For this review, take the finished solid that the model builds, in its own axes (mm). Coordinates: 2 decimals unless noted, no trailing zeros. Order: outer loops, then holes, each group sorted by start corner. A loop starts at its lowest first (then second) coordinate and runs counter-clockwise, first axis right, second up. Notation, with made-up numbers: (45.25, -16) -> (92.25, -16) arc R17 cw to (92.25, -7) -> close; hole circle Ø2 at (-13.5, 9.25). An arc over 180 degrees is marked (long way). Answer as a JSON object with one key per item and string values. Group by question number.
1) Wall thickness on L1, parallel to Y at x = 218, z = 0.9; L2, parallel to Y at x = 115, z = 1.25; L3, parallel to Y at x = 76.5, z = 1.25: over which ranges is each line inside the solid? List them lowest first.
2) Add section A-A, the plane y = 203.5. Write out the cut boundary in (x, z).
3) For pin 1 (3.5 mm diameter, centred on x = 111, y = 10.5, fed in from +Z), flat-tipped, find the tip position at first contact; note if it passes through.
4) Add section B-B, the plane z = 1.05. Count the separate pieces of the cut face and the enclosed holes in it, then the cut area to 3 significant figures.
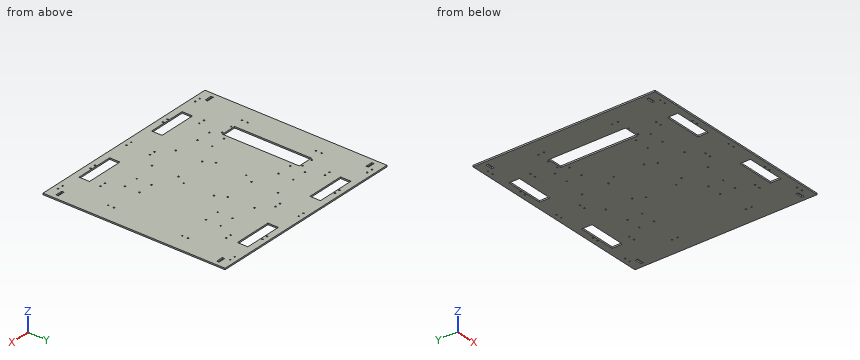
from build123d import *

# Parameters (mm, degrees)
SKETCH_1_W          = 424
SKETCH_1_H          = 384
SKETCH_1_W_2        = 80
SKETCH_1_H_2        = 22
EXTRUDE_1_DEPTH     = 3
SKETCH_2_R          = 1.5
SKETCH_2_W          = 32
SKETCH_2_H          = 162
CUT_EXTRUDE_1_DEPTH = 573.049823005
SKETCH_3_R          = 1.5
CUT_EXTRUDE_2_DEPTH = 573.049823005
SKETCH_4_R          = 1.5
CUT_EXTRUDE_3_DEPTH = 573.049823005
SKETCH_5_W          = 15
SKETCH_5_H          = 5
CUT_EXTRUDE_4_DEPTH = 573.049823005
SKETCH_6_R          = 1.5
CUT_EXTRUDE_5_DEPTH = 573.049823005


with BuildPart() as part:
    # 草图1 → 凸台-拉伸1 (new body)
    with BuildSketch(Plane.XY):
        with Locations((212, 192)):
            Rectangle(SKETCH_1_W, SKETCH_1_H)
        with Locations((307, 359)):
            Rectangle(SKETCH_1_W_2, SKETCH_1_H_2, mode=Mode.SUBTRACT)
        with Locations((117, 359)):
            Rectangle(SKETCH_1_W_2, SKETCH_1_H_2, mode=Mode.SUBTRACT)
        with Locations((307, 25)):
            Rectangle(SKETCH_1_W_2, SKETCH_1_H_2, mode=Mode.SUBTRACT)
        with Locations((117, 25)):
            Rectangle(SKETCH_1_W_2, SKETCH_1_H_2, mode=Mode.SUBTRACT)
    extrude(amount=EXTRUDE_1_DEPTH)

    # 草图2 → 切除-拉伸1 (cut, through all)
    with BuildSketch(Plane.XY.offset(3)):
        with Locations((64, 277)):
            Circle(SKETCH_2_R)
        with Locations((88, 277)):
            Circle(SKETCH_2_R)
        with Locations(Location((88, 107, 0), (0, 0, 180))):
            Circle(SKETCH_2_R)
        with Locations(Location((64, 107, 0), (0, 0, 180))):
            Circle(SKETCH_2_R)
        with Locations((76, 192)):
            Rectangle(SKETCH_2_W, SKETCH_2_H)
    extrude(amount=-CUT_EXTRUDE_1_DEPTH, mode=Mode.SUBTRACT)

    # 草图3 → 切除-拉伸2 (cut, through all)
    with BuildSketch(Plane.XY.offset(3)):
        with Locations((101.5, 293)):
            Circle(SKETCH_3_R)
        with Locations((132.5, 293)):
            Circle(SKETCH_3_R)
        with Locations((101.5, 262)):
            Circle(SKETCH_3_R)
        with Locations((132.5, 262)):
            Circle(SKETCH_3_R)
        with Locations(Location((322.5, 262, 0), (0, 0, 180))):
            Circle(SKETCH_3_R)
        with Locations(Location((291.5, 262, 0), (0, 0, 180))):
            Circle(SKETCH_3_R)
        with Locations(Location((291.5, 293, 0), (0, 0, 180))):
            Circle(SKETCH_3_R)
        with Locations(Location((322.5, 293, 0), (0, 0, 180))):
            Circle(SKETCH_3_R)
        with Locations((291.5, 122)):
            Circle(SKETCH_3_R)
        with Locations((322.5, 122)):
            Circle(SKETCH_3_R)
        with Locations((322.5, 91)):
            Circle(SKETCH_3_R)
        with Locations((291.5, 91)):
            Circle(SKETCH_3_R)
        with Locations(Location((101.5, 122, 0), (0, 0, 180))):
            Circle(SKETCH_3_R)
        with Locations(Location((132.5, 122, 0), (0, 0, 180))):
            Circle(SKETCH_3_R)
        with Locations(Location((132.5, 91, 0), (0, 0, 180))):
            Circle(SKETCH_3_R)
        with Locations(Location((101.5, 91, 0), (0, 0, 180))):
            Circle(SKETCH_3_R)
    extrude(amount=-CUT_EXTRUDE_2_DEPTH, mode=Mode.SUBTRACT)

    # 草图4 → 切除-拉伸3 (cut, through all)
    with BuildSketch(Plane.XY.offset(3)):
        with Locations((218, 10.5)):
            Circle(SKETCH_4_R)
        with Locations((301, 10.5)):
            Circle(SKETCH_4_R)
        with Locations((313, 10.5)):
            Circle(SKETCH_4_R)
        with Locations((385.5, 10.5)):
            Circle(SKETCH_4_R)
        with Locations((397.5, 10.5)):
            Circle(SKETCH_4_R)
        with Locations((218, 59.5)):
            Circle(SKETCH_4_R)
        with Locations((335.5, 59.5)):
            Circle(SKETCH_4_R)
        with Locations((347.5, 59.5)):
            Circle(SKETCH_4_R)
        with Locations((387, 108)):
            Circle(SKETCH_4_R)
        with Locations((387, 120)):
            Circle(SKETCH_4_R)
        with Locations(Location((387, 276, 0), (0, 0, 180))):
            Circle(SKETCH_4_R)
        with Locations(Location((387, 264, 0), (0, 0, 180))):
            Circle(SKETCH_4_R)
        with Locations(Location((301, 373.5, 0), (0, 0, 180))):
            Circle(SKETCH_4_R)
        with Locations(Location((313, 373.5, 0), (0, 0, 180))):
            Circle(SKETCH_4_R)
        with Locations(Location((397.5, 373.5, 0), (0, 0, 180))):
            Circle(SKETCH_4_R)
        with Locations(Location((385.5, 373.5, 0), (0, 0, 180))):
            Circle(SKETCH_4_R)
        with Locations(Location((347.5, 324.5, 0), (0, 0, 180))):
            Circle(SKETCH_4_R)
        with Locations(Location((335.5, 324.5, 0), (0, 0, 180))):
            Circle(SKETCH_4_R)
        with Locations(Location((218, 373.5, 0), (0, 0, 180))):
            Circle(SKETCH_4_R)
        with Locations(Location((206, 59.5, 0), (0, 0, 180))):
            Circle(SKETCH_4_R)
        with Locations(Location((206, 10.5, 0), (0, 0, 180))):
            Circle(SKETCH_4_R)
        with Locations(Location((111, 10.5, 0), (0, 0, 180))):
            Circle(SKETCH_4_R)
        with Locations(Location((123, 10.5, 0), (0, 0, 180))):
            Circle(SKETCH_4_R)
        with Locations(Location((26.5, 10.5, 0), (0, 0, 180))):
            Circle(SKETCH_4_R)
        with Locations(Location((38.5, 10.5, 0), (0, 0, 180))):
            Circle(SKETCH_4_R)
        with Locations(Location((76.5, 59.5, 0), (0, 0, 180))):
            Circle(SKETCH_4_R)
        with Locations(Location((88.5, 59.5, 0), (0, 0, 180))):
            Circle(SKETCH_4_R)
        with Locations(Location((37, 108, 0), (0, 0, 180))):
            Circle(SKETCH_4_R)
        with Locations(Location((37, 120, 0), (0, 0, 180))):
            Circle(SKETCH_4_R)
        with Locations((37, 264)):
            Circle(SKETCH_4_R)
        with Locations((37, 276)):
            Circle(SKETCH_4_R)
        with Locations((26.5, 373.5)):
            Circle(SKETCH_4_R)
        with Locations((38.5, 373.5)):
            Circle(SKETCH_4_R)
        with Locations((76.5, 324.5)):
            Circle(SKETCH_4_R)
        with Locations((88.5, 324.5)):
            Circle(SKETCH_4_R)
        with Locations((111, 373.5)):
            Circle(SKETCH_4_R)
        with Locations((123, 373.5)):
            Circle(SKETCH_4_R)
        with Locations((206, 373.5)):
            Circle(SKETCH_4_R)
        with Locations((206, 324.5)):
            Circle(SKETCH_4_R)
        with Locations(Location((218, 324.5, 0), (0, 0, 180))):
            Circle(SKETCH_4_R)
    extrude(amount=-CUT_EXTRUDE_3_DEPTH, mode=Mode.SUBTRACT)

    # 草图5 → 切除-拉伸4 (cut, through all)
    with BuildSketch(Plane.XY.offset(3)):
        with Locations((16.5, 361.5)):
            Rectangle(SKETCH_5_W, SKETCH_5_H)
        with Locations((407.5, 361.5)):
            Rectangle(SKETCH_5_W, SKETCH_5_H)
        with Locations((407.5, 22.5)):
            Rectangle(SKETCH_5_W, SKETCH_5_H)
        with Locations((16.5, 22.5)):
            Rectangle(SKETCH_5_W, SKETCH_5_H)
    extrude(amount=-CUT_EXTRUDE_4_DEPTH, mode=Mode.SUBTRACT)

    # 草图6 → 切除-拉伸5 (cut, through all)
    with BuildSketch(Plane.XY.offset(3)):
        with Locations((170, 224)):
            Circle(SKETCH_6_R)
        with Locations((170, 160)):
            Circle(SKETCH_6_R)
        with Locations((254, 160)):
            Circle(SKETCH_6_R)
        with Locations((254, 224)):
            Circle(SKETCH_6_R)
        with Locations((181, 300)):
            Circle(SKETCH_6_R)
        with Locations((243, 300)):
            Circle(SKETCH_6_R)
        with Locations((243, 244)):
            Circle(SKETCH_6_R)
        with Locations((181, 244)):
            Circle(SKETCH_6_R)
        with Locations(Location((181, 140, 0), (0, 0, 180))):
            Circle(SKETCH_6_R)
        with Locations(Location((243, 140, 0), (0, 0, 180))):
            Circle(SKETCH_6_R)
        with Locations(Location((243, 84, 0), (0, 0, 180))):
            Circle(SKETCH_6_R)
        with Locations(Location((181, 84, 0), (0, 0, 180))):
            Circle(SKETCH_6_R)
    extrude(amount=-CUT_EXTRUDE_5_DEPTH, mode=Mode.SUBTRACT)


solid = part.part
Output values:
{
 "1": {"L1": "y = 0 to 9, 12 to 58, 61 to 323, 326 to 372, 375 to 384", "L2": "y = 0 to 14, 36 to 348, 370 to 384", "L3": "y = 0 to 58, 61 to 111, 273 to 323, 326 to 384"},
 "2": {"outline": "(0, 0) -> (60, 0) -> (60, 3) -> (0, 3) -> close; (92, 0) -> (424, 0) -> (424, 3) -> (92, 3) -> close"},
 "3": {"pin 1": "stops at z = 3"},
 "4": {"separate pieces": "1", "enclosed holes": "81", "area": "150,000 mm²"}
}
